The listing builds one solid part. Answer for the finished solid, in the listing's coordinates (mm). Face numbers are marked on the shaded views. A direction names the side the tool comes from. Give positions to 0.01 mm unless a question says otherwise; leave off trailing zeros. Write each loop counter-clockwise with the first axis right and the second up, starting at its lowest first coordinate (ties: lowest second). Pieces come first, ordered by that corner, then holes.
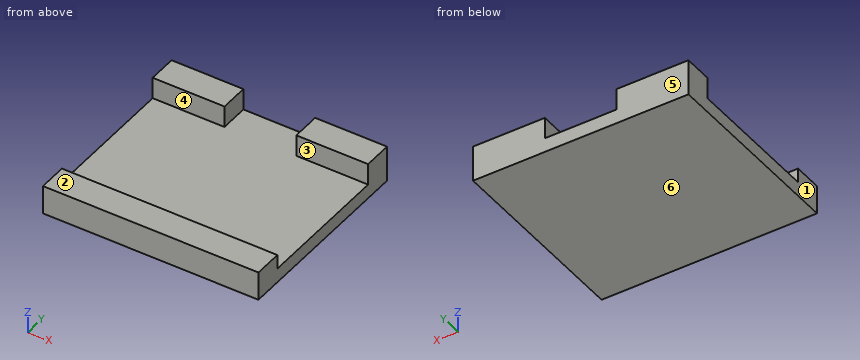
```python
from build123d import *

# Parameters (mm, degrees)
SKETCH1_W           = 30
SKETCH1_H           = 4
SKETCH1_H_2         = 19.2
BOSS_EXTRUDE1_DEPTH = 2
SKETCH1_4_W         = 30
SKETCH1_4_H         = 4
BOSS_EXTRUDE2_DEPTH = 2
SKETCH1_5_W         = 30
SKETCH1_5_H         = 4
BOSS_EXTRUDE3_DEPTH = 3
CUT_EXTRUDE1_REACH  = 6
SKETCH3_W           = 10
SKETCH3_H           = 3


with BuildPart() as part:
    # Sketch1 → Boss-Extrude1 (new body)
    with BuildSketch(Plane.XY):
        with Locations((0, 25.2)):
            Rectangle(SKETCH1_W, SKETCH1_H)
        with Locations((0, 13.6)):
            Rectangle(SKETCH1_W, SKETCH1_H_2)
        with Locations((0, 2)):
            Rectangle(SKETCH1_W, SKETCH1_H)
    extrude(amount=-BOSS_EXTRUDE1_DEPTH)

    # Sketch1_4 → Boss-Extrude2 (add)
    with BuildSketch(Plane.XY):
        with Locations((0, 2)):
            Rectangle(SKETCH1_4_W, SKETCH1_4_H)
    extrude(amount=BOSS_EXTRUDE2_DEPTH)

    # Sketch1_5 → Boss-Extrude3 (add)
    with BuildSketch(Plane.XY):
        with Locations((0, 25.2)):
            Rectangle(SKETCH1_5_W, SKETCH1_5_H)
    extrude(amount=BOSS_EXTRUDE3_DEPTH)

    # Sketch3 → Cut-Extrude1 (cut, up to next)
    with BuildSketch(Plane.XZ.offset(-23.2), mode=Mode.PRIVATE) as cut_extrude1_sk1:
        with Locations((0, 1.5)):
            Rectangle(SKETCH3_W, SKETCH3_H)
    cut_extrude1_tool1 = extrude(cut_extrude1_sk1.sketch, amount=-CUT_EXTRUDE1_REACH, mode=Mode.PRIVATE) & part.part
    add(cut_extrude1_tool1.solids().sort_by_distance((0, 23.2, 1.5))[0], mode=Mode.SUBTRACT)


solid = part.part
```
Item 1: A cutting plane is placed at A-A, the plane z = 0.7. Give the vertices of the cut face in (x, y).
Conclusion:
outline: (-15, 0) - (15, 0) - (15, 4) - (-15, 4) - close; (-15, 23.2) - (-5, 23.2) - (-5, 27.2) - (-15, 27.2) - close; (5, 23.2) - (15, 23.2) - (15, 27.2) - (5, 27.2) - close
Item 2: Consider probe 1 along Y at (x, z) = (8.5, 0.55); probe 2 along Z at (x, y) = (13.75, 1.5); probe 3 along Y at (x, z) = (-7.25, 2.8). Determine where each line is inside the solid, lowest interval first.
Conclusion:
probe 1: y = 0 to 4, 23.2 to 27.2
probe 2: z = -2 to 2
probe 3: y = 23.2 to 27.2
Item 3: A cutting plane is placed at D-D, the plane x = 7.5. Give the vertices of the cut face in (y, z), plus the area to 3 significant figures.
Conclusion:
outline: (0, -2) - (27.2, -2) - (27.2, 3) - (23.2, 3) - (23.2, 0) - (4, 0) - (4, 2) - (0, 2) - close
area: 74.4 mm2
Item 4: Determine the mould class of the marked faces 4, 5 and 6 for opening direction Y: pulls with the +Y half, pulls with the -Y half, needs draft (parallel to the pull), parting line crosses it, or undercut.
Conclusion:
face 4: undercut
face 5: pulls with the +Y half
face 6: needs draft
Item 5: Which of the six approach directions +Z, -Z, +X, -X, +Y, -Y give full straight-line access (tool end or side, diameter ignored) to the marked faces 1, 2 and 3?
Conclusion:
face 1: +Z, -Z, -X, +Y, -Y
face 2: +Z, +X, -X, -Y
face 3: +Z, +X, -X
Item 6: Each of these flat-tipped pins is pushed along its axis until it touches: P1, Ø4.5, axis at x = 1.5, y = 2.5, coming from the +Z side; P2, Ø1, axis at x = -2, z = 1.5, coming from the +Y side; P3, Ø4, axis at x = 8.5, y = 10, coming from the +Z side. Where does it stop, or does it pass through?
Conclusion:
P1: stops at z = 2
P2: stops at y = 4
P3: stops at z = 0
Item 7: A cutting plane is placed at C-C, the plane y = 17.5. Give the vertices of the cut face in (x, z), plus the area to 3 significant figures.
Conclusion:
outline: (-15, -2) - (15, -2) - (15, 0) - (-15, 0) - close
area: 60.0 mm2
Item 8: A cutting plane is placed at B-B, the plane x = -4. Give the vertices of the cut face in (y, z), plus the area to 3 significant figures.
Conclusion:
outline: (0, -2) - (27.2, -2) - (27.2, 0) - (4, 0) - (4, 2) - (0, 2) - close
area: 62.4 mm2
